Work out the finished part from the listing and answer in its coordinate system (mm). A direction names the side the tool comes from. Round coordinates to 2 decimals unless told otherwise and drop trailing zeros. Order: outer loops, then holes, each group sorted by start corner. A loop starts at its lowest first (then second) coordinate and runs counter-clockwise, first axis right, second up.
from build123d import *

# Parameters (mm, degrees)
CYLINDER006_R             = 26.7
CYLINDER006_DEPTH         = 7.25
CYLINDER007_R             = 4.5
CYLINDER007_DEPTH         = 32
CYLINDER005_R             = 26.7
CYLINDER005_DEPTH         = 7.25
CYLINDER004_R             = 32
CYLINDER004_DEPTH         = 6.5
CYLINDER010_R             = 11.2
CYLINDER010_DEPTH         = 7
CYLINDER009_R             = 4.5
CYLINDER009_DEPTH         = 32
CYLINDER001_R             = 26.5
CYLINDER001_DEPTH         = 7.25
CYLINDER_R                = 32
CYLINDER_DEPTH            = 5.75
CYLINDER011_R             = 11.2
CYLINDER011_DEPTH         = 7
CYLINDER008_R             = 4.5
CYLINDER008_DEPTH         = 32
CYLINDER003_R             = 26.5
CYLINDER003_DEPTH         = 7.25
CYLINDER002_R             = 32
CYLINDER002_DEPTH         = 5.75
FUSION001_PLACEMENT_ANGLE = 180


with BuildPart() as cylinder006:
    # Cylinder006 → Cylinder006 (new body)
    with BuildSketch(Plane.XY.offset(7.75)):
        Circle(CYLINDER006_R)
    extrude(amount=CYLINDER006_DEPTH)


with BuildPart() as cylinder007:
    # Cylinder007 → Cylinder007 (new body)
    with BuildSketch(Plane.XY):
        Circle(CYLINDER007_R)
    extrude(amount=CYLINDER007_DEPTH)


with BuildPart() as fusion003:
    # Cylinder005 → Cylinder005 (new body)
    with BuildSketch(Plane.XY.offset(17)):
        Circle(CYLINDER005_R)
    extrude(amount=CYLINDER005_DEPTH)

    # Fusion003: union Cylinder006, Cylinder007
    add(cylinder006.part)
    add(cylinder007.part)


with BuildPart() as cone002:
    # Cone002 → Cone002 (revolve)
    with BuildSketch(Plane(origin=(0, 0, 8.5), x_dir=(1, 0, 0), z_dir=(0, -1, 0))):
        Polygon((0, 0), (32, 0), (30, 2), (0, 2), align=None)
    revolve(axis=Axis((0, 0, 8.5), (0, 0, 1)))


with BuildPart() as cone003:
    # Cone003 → Cone003 (revolve)
    with BuildSketch(Plane.XZ):
        Polygon((0, 0), (30, 0), (32, 2), (0, 2), align=None)
    revolve(axis=Axis((0, 0, 0), (0, 0, 1)))


with BuildPart() as cut:
    # Cylinder004 → Cylinder004 (new body)
    with BuildSketch(Plane.XY.offset(2)):
        Circle(CYLINDER004_R)
    extrude(amount=CYLINDER004_DEPTH)

    # Fusion002: union Cone002, Cone003
    add(cone002.part)
    add(cone003.part)


with BuildPart() as cut_1:
    # Fusion002 placement: moved
    add(cut.part.moved(Location((0, 0, 10.75))))

    # Cut: cut Fusion003
    add(fusion003.part, mode=Mode.SUBTRACT)


with BuildPart() as cylinder010:
    # Cylinder010 → Cylinder010 (new body)
    with BuildSketch(Plane.XY):
        Circle(CYLINDER010_R)
    extrude(amount=CYLINDER010_DEPTH)


with BuildPart() as cylinder009:
    # Cylinder009 → Cylinder009 (new body)
    with BuildSketch(Plane.XY):
        Circle(CYLINDER009_R)
    extrude(amount=CYLINDER009_DEPTH)


with BuildPart() as cone:
    # Cone → Cone (revolve)
    with BuildSketch(Plane(origin=(0, 0, 5.75), x_dir=(1, 0, 0), z_dir=(0, -1, 0))):
        Polygon((0, 0), (32, 0), (30, 2), (0, 2), align=None)
    revolve(axis=Axis((0, 0, 5.75), (0, 0, 1)))


with BuildPart() as cylinder001:
    # Cylinder001 → Cylinder001 (new body)
    with BuildSketch(Plane.XY.offset(7.75)):
        Circle(CYLINDER001_R)
    extrude(amount=CYLINDER001_DEPTH)


with BuildPart() as cut003:
    # Cylinder → Cylinder (new body)
    with BuildSketch(Plane.XY):
        Circle(CYLINDER_R)
    extrude(amount=CYLINDER_DEPTH)

    # Fusion: union Cone, Cylinder001
    add(cone.part)
    add(cylinder001.part)

    # Cut002: cut Cylinder009
    add(cylinder009.part, mode=Mode.SUBTRACT)

    # Cut003: cut Cylinder010
    add(cylinder010.part, mode=Mode.SUBTRACT)


with BuildPart() as cylinder011:
    # Cylinder011 → Cylinder011 (new body)
    with BuildSketch(Plane.XY.offset(25)):
        Circle(CYLINDER011_R)
    extrude(amount=CYLINDER011_DEPTH)


with BuildPart() as cylinder008:
    # Cylinder008 → Cylinder008 (new body)
    with BuildSketch(Plane.XY):
        Circle(CYLINDER008_R)
    extrude(amount=CYLINDER008_DEPTH)


with BuildPart() as cone001:
    # Cone001 → Cone001 (revolve)
    with BuildSketch(Plane(origin=(0, 0, 5.75), x_dir=(1, 0, 0), z_dir=(0, -1, 0))):
        Polygon((0, 0), (32, 0), (30, 2), (0, 2), align=None)
    revolve(axis=Axis((0, 0, 5.75), (0, 0, 1)))


with BuildPart() as cylinder003:
    # Cylinder003 → Cylinder003 (new body)
    with BuildSketch(Plane.XY.offset(7.75)):
        Circle(CYLINDER003_R)
    extrude(amount=CYLINDER003_DEPTH)


with BuildPart() as fusion004:
    # Cylinder002 → Cylinder002 (new body)
    with BuildSketch(Plane.XY):
        Circle(CYLINDER002_R)
    extrude(amount=CYLINDER002_DEPTH)

    # Fusion001: union Cone001, Cylinder003
    add(cone001.part)
    add(cylinder003.part)


with BuildPart() as fusion004_1:
    # Fusion001 placement: moved
    add(fusion004.part.moved(Location((0, 0, 32))).rotate(Axis((0, 0, 32), (1, 0, 0)), FUSION001_PLACEMENT_ANGLE))

    # Cut001: cut Cylinder008
    add(cylinder008.part, mode=Mode.SUBTRACT)

    # Cut004: cut Cylinder011
    add(cylinder011.part, mode=Mode.SUBTRACT)

    # Fusion004: union Cut, Cut003
    add(cut_1.part)
    add(cut003.part)


solid = fusion004_1.part
Item 1: A tool of negligible diameter and unlimited length cuts with its end or side. For faces 4 (the face through (25.467, 8.02, 19.095)), 5 (the face through (-11.19, 0.49, 3.45)), 6 (the face through (-11.19, 0.49, 28.45)), from which of +Z, -Z, +X, -X, +Y, -Y can it reach the whole face along a straight path? Write none if from no direction.
Item 2: Find the intervals of material crossed by line 1 along Y through (x, z) = (0, 13); line 2 along Y through (x, z) = (18, 18); line 3 along Y through (x, z) = (0, 30.25), in increasing order.
Item 3: Find section A-A (z = 14). Write down the section's boundary in (x, y).
Item 4: Given pin 1 (2 mm diameter, centred on y = 13.5, z = 20.5, fed in from +X); pin 2 (5 mm diameter, centred on y = -7.5, z = 5.5, fed in from -X); pin 3 (11 mm diameter, centred on x = 1.5, y = 2.5, fed in from -Z), each flat-ended and moving along its own axis, determine where each tip first touches the part or whether it passes through.
Item 5: For a pull along X with two mould halves and no side action, classify faces 1 (the face through (14.246, -22.345, 20.676)), 2 (the face through (-6.94, -31.24, 15.95)), 3 (the face through (14, 0, 32)) as released by +X, released by -X, zero draft, split by the parting line, or undercut.
Model answer:
1. face 4: none
1. face 5: -Z
1. face 6: +Z
2. line 1: y = -32 to -26.7, -26.5 to -4.5, 4.5 to 26.5, 26.7 to 32
2. line 2: y = -26.46 to -19.72, -19.45 to 19.45, 19.72 to 26.46
2. line 3: y = -32 to -11.2, 11.2 to 32
3. outline: circle Ø64 at (0, 0); circle Ø53 at (0, 0); hole circle Ø53.4 at (0, 0); hole circle Ø9 at (0, 0)
4. pin 1: stops at x = 28.83
4. pin 2: stops at x = -31.61
4. pin 3: stops at z = 7
5. face 1: undercut
5. face 2: split by the parting line
5. face 3: zero draft
